from build123d import *

# Parameters (mm, degrees)
SKETCH_R           = 4.125
PAD_DEPTH          = 76
SKETCH001_R        = 1.5
POCKET_DEPTH       = 5
POLARPATTERN_COUNT = 3
FILLET_R           = 1
FILLET001_R        = 0.2


with BuildPart() as part:
    # Sketch → Pad (new body)
    with BuildSketch(Plane.XY):
        Polygon((-11, -6.350853), (-1, 10.969655), (-2, 13.669655), (-9, 16.669655), (-10, 17.669655), (10, 17.669655), (9, 16.669655), (2, 13.669655), (1, 10.969655), (11, -6.350853), align=None)
        Circle(SKETCH_R, mode=Mode.SUBTRACT)
    extrude(amount=PAD_DEPTH)

    # Sketch001 → Pocket (cut)
    with BuildSketch(Plane.XZ.offset(6.350853)):
        with Locations((0, 38)):
            Circle(SKETCH001_R)
    pocket = extrude(amount=-POCKET_DEPTH, mode=Mode.SUBTRACT)

    # PolarPattern: Pocket ×3 about axis
    polarpattern_axis = Axis((0, 0, 0), (0, 0, 1))
    for i in range(1, POLARPATTERN_COUNT):
        add(pocket.rotate(polarpattern_axis, i * 360 / POLARPATTERN_COUNT), mode=Mode.SUBTRACT)

    # Fillet
    fillet_edges = [part.edges().sort_by_distance(p)[0] for p in [
        (11, -6.350853, 38),
        (-11, -6.350853, 38),
    ]]
    fillet(fillet_edges, radius=FILLET_R)

    # Fillet001
    fillet001_edges = [part.edges().sort_by_distance(p)[0] for p in [
        (10, 17.669655, 38),
        (-10, 17.669655, 38),
    ]]
    fillet(fillet001_edges, radius=FILLET001_R)


solid = part.part
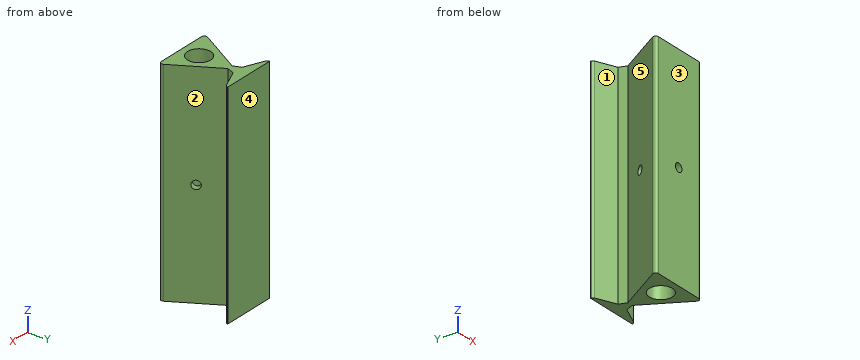
Input: part model. Units: mm. Frame: model coordinates. Face numbers are marked on the shaded views. A direction names the side the tool comes from. Round coordinates to 2 decimals unless told otherwise and drop trailing zeros. Loops run counter-clockwise (first coordinate to the right, second up) from the corner with the lowest first, then second, coordinate; pieces in that order, holes last. Notation, with made-up numbers: M 42,-18 L 86,-18 A12 ccw 86,-1 Z; hole C 45,48.25 d7. An arc over 180 degrees is marked long. Answer as CSV lines item,"result". Start each with the question number.
(1) Line query: line 1 (Z direction, x = 0, y = -5.25); line 2 (Y direction, x = 3.5, z = 21); line 3 (Y direction, x = 0, z = 44) (3 decimals). Output: solid intervals per line, ascending. Write a range as [from, to].
(2) Section C-C, the plane x = 8.25. Output: boundary loops of the cut face in (y, z), plus the area to 3 significant figures.
(3) Section D-D, the plane z = 38. Output: boundary loops of the cut face in (x, y) (3 decimals).
(4) Draft query along Y for the marked faces 3, 4 and 5. Return one class per face: released by +Y, released by -Y, zero draft, split by the parting line, or undercut.
(5) Section A-A, the plane x = 0. Output: boundary loops of the cut face in (y, z) (3 decimals), plus the area to 3 significant figures.
(6) Section B-B, the plane z = 28. Output: boundary loops of the cut face in (x, y) (3 decimals), plus the area to 3 significant figures.
(7) Reachability of the marked faces 1 and 2 from +Z, -Z, +X, -X, +Y, -Y: full face, straight path, thin tool, end or side. Return the list, or none.
(8) First-contact query: pin 1 (4 mm diameter, centred on y = 3.5, z = 21, fed in from +X); pin 2 (3 mm diameter, centred on x = -0.5, y = 12.5, fed in from -Z); pin 3 (2 mm diameter, centred on y = 10.5, z = 51, fed in from -X). Flat tips, straight axial feed; report the tip coordinate or a pass-through.
Values found:
1,line 1,"z = [0, 36.5], [39.5, 76]"
1,line 2,"y = [-6.35, -2.18], [2.18, 6.64], [14.31, 17.67]"
1,line 3,"y = [-6.351, -4.125], [4.125, 17.67]"
2,outline,"M -6.35,0 L -1.59,0 L -1.59,76 L -6.35,76 Z; M 16.35,0 L 17.67,0 L 17.67,76 L 16.35,76 Z"
2,area,"462 mm²"
3,outline,"M -10.134,-4.851 A1 ccw -9.268,-6.351 L -1.5,-6.351 L -1.5,-3.843 A4.125 cw -4.078,0.622 L -6.25,1.876 Z; M -9.659,17.328 L -9,16.67 L -2,13.67 L -1,10.97 L -4.75,4.474 L -2.578,3.22 A4.125 cw 2.578,3.22 L 4.75,4.474 L 1,10.97 L 2,13.67 L 9,16.67 L 9.659,17.328 A0.2 ccw 9.517,17.67 L -9.517,17.67 A0.2 ccw Z; M 1.5,-6.351 L 9.268,-6.351 A1 ccw 10.134,-4.851 L 6.25,1.876 L 4.078,0.622 A4.125 cw 1.5,-3.843 Z"
4,face 3,"released by -Y"
4,face 4,"released by +Y"
4,face 5,"undercut"
5,outline,"M -6.351,0 L -4.125,0 L -4.125,36.5 L -6.351,36.5 Z; M -6.351,39.5 L -4.125,39.5 L -4.125,76 L -6.351,76 Z; M 4.125,0 L 17.67,0 L 17.67,76 L 4.125,76 Z"
5,area,"1,190 mm²"
6,outline,"M -10.134,-4.851 A1 ccw -9.268,-6.351 L 9.268,-6.351 A1 ccw 10.134,-4.851 L 1,10.97 L 2,13.67 L 9,16.67 L 9.659,17.328 A0.2 ccw 9.517,17.67 L -9.517,17.67 A0.2 ccw -9.659,17.328 L -9,16.67 L -2,13.67 L -1,10.97 Z; hole C 0,0 d8.25"
6,area,"213 mm²"
7,face 1,"+Z, -Z, -X"
7,face 2,"+Z, -Z, +X"
8,pin 1,"stops at x = 6.47"
8,pin 2,"stops at z = 0"
8,pin 3,"stops at x = -1.85"
